Check sheet for the drawn part. Datum: minimum x, y, z corner. Units: mm. A direction names the side the tool comes from. Coordinates: 2 decimals unless noted, no trailing zeros. Order: outer loops, then holes, each group sorted by start corner. A loop starts at its lowest first (then second) coordinate and runs counter-clockwise, first axis right, second up.
1. Thickness scan on line 1 (X direction, y = 2.75, z = 24); line 2 (X direction, y = 9.5, z = 22); line 3 (X direction, y = 8, z = 24). Record the ranges inside material, lowest first.
2. Cross-section at D-D (y = 6.25). Enter the section's corners in (x, z), then the cut area to 3 significant figures.
3. Cross-section at B-B (y = 1.25). Enter the section's corners in (x, z).
4. Cross-section at A-A (x = 24). Enter the section's corners in (y, z), then the cut area to 3 significant figures.
5. Cross-section at C-C (z = 24). Enter the section's corners in (x, y), then the cut area to 3 significant figures.
6. Set-up check for the marked faces 1, 2 and 3: record each of +Z, -Z, +X, -X, +Y, -Y from which the full face is reachable in a straight line by a thin tool's end or side.
7. Gauge pin test, flat ends, axial feed: pin 1 Ø3 at (x, z) = (5, 23.5) entering from +Y; pin 2 Ø6 at (x, y) = (25, 4) entering from -Z; pin 3 Ø3 at (y, z) = (3, 22.5) entering from +X; pin 4 Ø1.5 at (x, y) = (26.5, 9.5) entering from +Z. Record the tip position at first contact, or that the pin passes through.
8. Draft check along X on the marked faces 4, 5 and 6. Enter one of: released by +X, released by -X, zero draft, split by the parting line, or undercut.
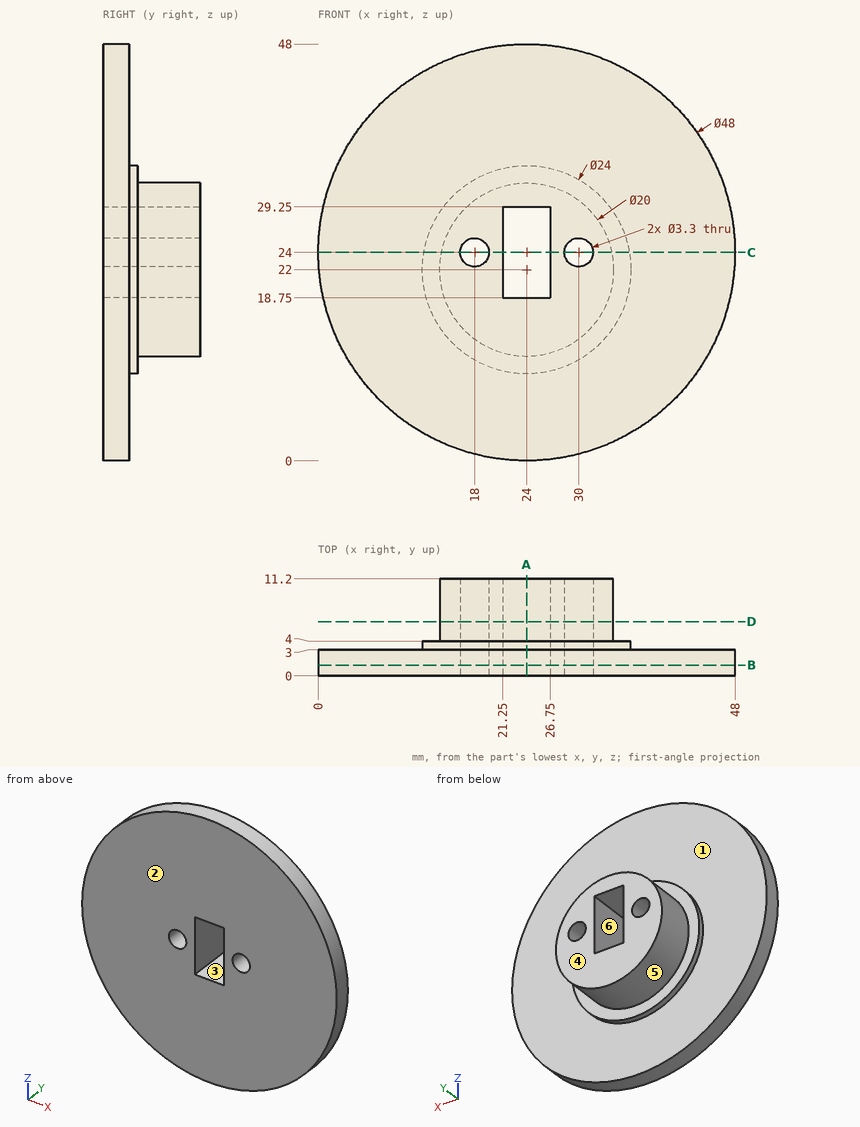
Data:
1. line 1: x = 0 to 16.35, 19.65 to 21.25, 26.75 to 28.35, 31.65 to 48
1. line 2: x = 14 to 21.25, 26.75 to 34
1. line 3: x = 14.2 to 16.35, 19.65 to 21.25, 26.75 to 28.35, 31.65 to 33.8
2. outline: circle Ø20 at (24, 22); hole circle Ø3.3 at (18, 24); hole (21.25, 18.75) - (26.75, 18.75) - (26.75, 29.25) - (21.25, 29.25) - close; hole circle Ø3.3 at (30, 24)
2. area: 239 mm2
3. outline: circle Ø48 at (24, 24); hole circle Ø3.3 at (18, 24); hole (21.25, 18.75) - (26.75, 18.75) - (26.75, 29.25) - (21.25, 29.25) - close; hole circle Ø3.3 at (30, 24)
4. outline: (0, 0) - (3, 0) - (3, 10) - (4, 10) - (4, 12) - (11.2, 12) - (11.2, 18.75) - (0, 18.75) - close; (0, 29.25) - (11.2, 29.25) - (11.2, 32) - (4, 32) - (4, 34) - (3, 34) - (3, 48) - (0, 48) - close
4. area: 194 mm2
5. outline: (0, 0) - (16.35, 0) - (16.35, 11.2) - (14.2, 11.2) - (14.2, 4) - (12.17, 4) - (12.17, 3) - (0, 3) - close; (19.65, 0) - (21.25, 0) - (21.25, 11.2) - (19.65, 11.2) - close; (26.75, 0) - (28.35, 0) - (28.35, 11.2) - (26.75, 11.2) - close; (31.65, 0) - (48, 0) - (48, 3) - (35.83, 3) - (35.83, 4) - (33.8, 4) - (33.8, 11.2) - (31.65, 11.2) - close
5. area: 173 mm2
6. face 1: +Y
6. face 2: +Z, -Z, +X, -X, -Y
6. face 3: +Y, -Y
7. pin 1: stops at y = 3
7. pin 2: stops at z = 0
7. pin 3: stops at x = 48
7. pin 4: stops at z = 31.85
8. face 4: zero draft
8. face 5: split by the parting line
8. face 6: undercut
